Can you work these out from the model? Positions are in its coordinate system, mm. Face numbers are marked on the shaded views. A direction names the side the tool comes from. Coordinates: 2 decimals unless noted, no trailing zeros. Order: outer loops, then holes, each group sorted by start corner. A loop starts at its lowest first (then second) coordinate and runs counter-clockwise, first axis right, second up. Notation, with made-up numbers: (-4, 68) -> (17, 68) arc R12 ccw to (17, 75) -> close; hole circle Ø2 at (61, 88). An arc over 180 degrees is marked (long way). Write item = value, one per line.
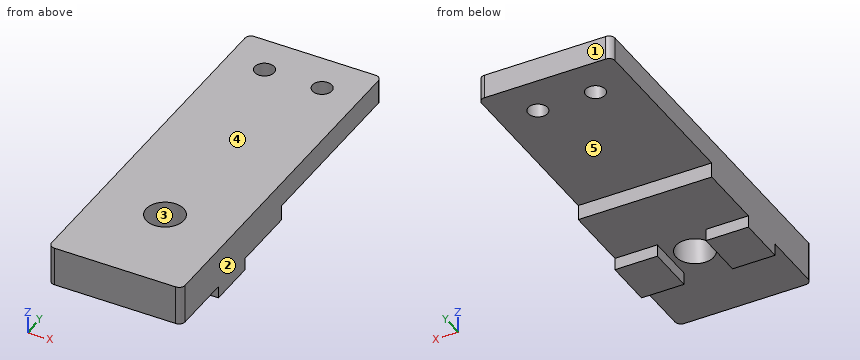
```python
from build123d import *

# Parameters (mm, degrees)
SKETCH_W        = 22
SKETCH_H        = 60
PAD_DEPTH       = 4
SKETCH001_W     = 22
SKETCH001_H     = 30
PAD001_DEPTH    = 2.5
SKETCH002_W     = 7
SKETCH002_H     = 8
PAD002_DEPTH    = 2
SKETCH003_R     = 3.1
POCKET_DEPTH    = 6.501
SKETCH004_R     = 1.6
POCKET001_DEPTH = 8.501
FILLET_R        = 1


with BuildPart() as part:
    # Sketch → Pad (new body)
    with BuildSketch(Plane.XY):
        with Locations((0, 15)):
            Rectangle(SKETCH_W, SKETCH_H)
    extrude(amount=PAD_DEPTH)

    # Sketch001 (on Face5 of Pad) → Pad001 (join)
    with BuildSketch(Plane(origin=(0, 0, 0), x_dir=(1, 0, 0), z_dir=(0, 0, -1))):
        Rectangle(SKETCH001_W, SKETCH001_H)
    extrude(amount=PAD001_DEPTH)

    # Sketch002 (on Face5 of Pad001) → Pad002 (join)
    with BuildSketch(Plane(origin=(0, 0, -2.5), x_dir=(1, 0, 0), z_dir=(0, 0, -1))):
        with Locations((-7.5, 0)):
            Rectangle(SKETCH002_W, SKETCH002_H)
        with Locations((7.5, 0)):
            Rectangle(SKETCH002_W, SKETCH002_H)
    extrude(amount=PAD002_DEPTH)

    # Sketch003 (on Face5 of Pad002) → Pocket (cut, through all)
    with BuildSketch(Plane(origin=(0, 0, -2.5), x_dir=(1, 0, 0), z_dir=(0, 0, -1))):
        Circle(SKETCH003_R)
    extrude(amount=-POCKET_DEPTH, mode=Mode.SUBTRACT)

    # Sketch004 (on Face5 of Pocket) → Pocket001 (cut, through all)
    with BuildSketch(Plane.XY.offset(4)):
        with Locations((-4.75, 38.5)):
            Circle(SKETCH004_R)
        with Locations((4.75, 38.5)):
            Circle(SKETCH004_R)
    extrude(amount=-POCKET001_DEPTH, mode=Mode.SUBTRACT)

    # Fillet
    fillet_edges = [part.edges().sort_by_distance(p)[0] for p in [
        (-11, -15, 0.75),
        (11, -15, 0.75),
        (-11, 45, 2),
        (11, 45, 2),
    ]]
    fillet(fillet_edges, radius=FILLET_R)


solid = part.part
```
Item 1: I want a section at C-C, the plane y = 0. Please give me the cut outline in (x, z), plus the area to 3 significant figures.
A:
outline = (-11, -4.5) -> (-4, -4.5) -> (-4, -2.5) -> (-3.1, -2.5) -> (-3.1, 4) -> (-11, 4) -> close; (3.1, -2.5) -> (4, -2.5) -> (4, -4.5) -> (11, -4.5) -> (11, 4) -> (3.1, 4) -> close
area = 131 mm2
Item 2: I want a section at D-D, the plane z = 1. Please give me the cut outline in (x, y).
A:
outline = (-11, -14) arc R1 ccw to (-10, -15) -> (10, -15) arc R1 ccw to (11, -14) -> (11, 44) arc R1 ccw to (10, 45) -> (-10, 45) arc R1 ccw to (-11, 44) -> close; hole circle Ø3.2 at (-4.75, 38.5); hole circle Ø6.2 at (0, 0); hole circle Ø3.2 at (4.75, 38.5)
Item 3: I'm going to push flat-ended pins straight in: P1, Ø2, axis at x = 8.5, z = -4, coming from the -Y side; P2, Ø0.6, axis at x = -7, z = -3.5, coming from the +Y side; P3, Ø4, axis at y = -8.5, z = -3.5, coming from the +X side; P4, Ø1.5, axis at x = 7.5, y = 20, coming from the -Z side. Where does each tip first touch, or does it pass through?
A:
P1 = -4
P2 = 4
P3 = 11
P4 = 0
Item 4: If we mould it in two halves opening along X, with no side actions, what happens to the marked faces 1, 2 and 3? For each: pulls with the +X half, pulls with the -X half, needs draft (parallel to the pull), parting line crosses it, or undercut.
A:
face_1 = needs draft
face_2 = pulls with the +X half
face_3 = undercut
Item 5: For the marked faces 4 and 5, which set-ups out of +Z, -Z, +X, -X, +Y, -Y let a thin tool reach every point of the face, with its end or its side?
A:
face_4 = +Z, +X, -X, +Y, -Y
face_5 = -Z, +X, -X, +Y
Item 6: I want a section at A-A, the plane y = 38.5. Please give me the cut outline in (x, z), plus the area to 3 significant figures.
A:
outline = (-11, 0) -> (-6.35, 0) -> (-6.35, 4) -> (-11, 4) -> close; (-3.15, 0) -> (3.15, 0) -> (3.15, 4) -> (-3.15, 4) -> close; (6.35, 0) -> (11, 0) -> (11, 4) -> (6.35, 4) -> close
area = 62.4 mm2
Item 7: I want a section at B-B, the plane x = 4.75. Please give me the cut outline in (y, z), plus the area to 3 significant figures.
A:
outline = (-15, -2.5) -> (-4, -2.5) -> (-4, -4.5) -> (4, -4.5) -> (4, -2.5) -> (15, -2.5) -> (15, 0) -> (36.9, 0) -> (36.9, 4) -> (-15, 4) -> close; (40.1, 0) -> (45, 0) -> (45, 4) -> (40.1, 4) -> close
area = 318 mm2
Item 8: If I drill on probe 1 along X at (y, z) = (0, 0.25); probe 2 along Y at (x, z) = (-4.75, 2.1); probe 3 along Z at (x, y) = (-1.25, 18), over which ranges is the centre line in solid material (lowest first)?
A:
probe_1 = -11 to -3.1, 3.1 to 11
probe_2 = -15 to 36.9, 40.1 to 45
probe_3 = 0 to 4
